```python
from build123d import *

# Parameters (mm, degrees)
F0_W      = 8
F0_H      = 5
F1_DEPTH  = 5
F2_R      = 0.75
F3_DEPTH  = 2
F4_W      = 4
F4_H      = 1.5
F5_DEPTH  = 23.5
F7_DEPTH  = 1.5
F8_W      = 1
F8_H      = 4
F9_DEPTH  = 30
F10_W     = 1
F10_H     = 2
F11_DEPTH = 1.5
F12_R     = 5
F13_DEPTH = 1
F15_ANGLE = 180
F16_R     = 0.49999
F17_R     = 0.5
F18_R     = 0.5


# Not quite as in the source:
# - a fillet or chamfer is up to 0.001 mm smaller than in the source, because OpenCascade refuses the exact size
# - a feature names something its author has since deleted; it is built from what else it names


with BuildPart() as f1:
    # F0 (on Front) → F1 (new body)
    with BuildSketch(Plane.XZ):
        Rectangle(F0_W, F0_H)
    extrude(amount=F1_DEPTH)

    # F2 (on face) → F3 (join)
    with BuildSketch(Plane.XZ.offset(5)):
        with Locations((-3, 1.5)):
            Circle(F2_R)
        with Locations((3, 1.5)):
            Circle(F2_R)
        with Locations((-3, -1.5)):
            Circle(F2_R)
        with Locations((3, -1.5)):
            Circle(F2_R)
    extrude(amount=F3_DEPTH)

    # F4 (on face) → F5 (join)
    with BuildSketch(Plane.XY.offset(2.5)):
        with Locations((0, -0.75)):
            Rectangle(F4_W, F4_H)
    extrude(amount=F5_DEPTH)

    # F6 (on face) → F7 (join)
    with BuildSketch(Plane(origin=(0, 0, 0), x_dir=(-1, 0, 0), z_dir=(0, 1, 0))):
        with BuildLine():
            ThreePointArc((2, 19.876524617), (4.5414755311, 21.8975815885), (5.5, 25))
            ThreePointArc((5.5, 25), (-3.1024184115, 29.5414755311), (-2, 19.876524617))
            Line((-2, 19.876524617), (-2, 26))
            Line((-2, 26), (2, 26))
            Line((2, 26), (2, 19.876524617))
        make_face()
        with BuildLine():
            Line((-2, 26), (-2, 19.876524617))
            ThreePointArc((-2, 19.876524617), (0, 19.5), (2, 19.876524617))
            Line((2, 19.876524617), (2, 26))
            Line((2, 26), (-2, 26))
        make_face()
    extrude(amount=-F7_DEPTH)

    # F8 (on face) → F9 (join)
    with BuildSketch(Plane.XZ.offset(1.5)):
        with Locations((0, 25)):
            Rectangle(F8_W, F8_H)
    extrude(amount=F9_DEPTH)

    # F10 (on face) → F11 (join)
    with BuildSketch(Plane.XZ.offset(31.5)):
        with Locations((0, 25)):
            Rectangle(F10_W, F10_H)
    extrude(amount=F11_DEPTH)

    # F12 (on face) → F13 (join)
    with BuildSketch(Plane(origin=(0, 0, 0), x_dir=(-1, 0, 0), z_dir=(0, 1, 0))):
        with Locations((0, 25)):
            Circle(F12_R)
    extrude(amount=F13_DEPTH)

    # F14 (on face) → F15 (revolve)
    with BuildSketch(Plane(origin=(0, 1, 0), x_dir=(-1, 0, 0), z_dir=(0, 1, 0))):
        with BuildLine():
            Line((0, 20), (0, 30))
            ThreePointArc((0, 30), (-5, 25), (0, 20))
        make_face()
    revolve(axis=Axis((0, 1, 25), (0, 0, 1)), revolution_arc=F15_ANGLE)

    # F16 (radius 0.5 in the source; OpenCascade refuses exactly that, so slightly less here)
    f16_edges = [f1.edges().sort_by_distance(p)[0] for p in [
        (-0.5, -16.5, 27),
        (0.5, -16.5, 27),
        (0.5, -16.5, 23),
        (-0.5, -16.5, 23),
    ]]
    fillet(f16_edges, radius=F16_R)

    # F17
    f17_edges = [f1.edges().sort_by_distance(p)[0] for p in [
        (-4, -2.5, 2.5),
        (-4, -2.5, -2.5),
        (4, -2.5, -2.5),
        (4, -2.5, 2.5),
    ]]
    fillet(f17_edges, radius=F17_R)

    # F18
    f18_edges = [f1.edges().sort_by_distance(p)[0] for p in [
        (-2, -1.5, 11.188262),
        (2, -1.5, 11.188262),
        (0, -1.5, 30.5),
    ]]
    fillet(f18_edges, radius=F18_R)


solid = f1.part
```
Model file for the job. Use its own axes, mm. A direction names the side the tool comes from. Coordinates: 2 decimals unless noted, no trailing zeros. Loops run counter-clockwise (first coordinate to the right, second up) from the corner with the lowest first, then second, coordinate; pieces in that order, holes last. Notation, with made-up numbers: (-3, 73) -> (20, 73) arc R23 ccw to (20, 84) -> close; hole circle Ø9 at (-22, 24.5). An arc over 180 degrees is marked (long way). Answer as a JSON object with one key per item and string values.
Q1. Pull direction Z, two halves, no side cores. Call faces 5 (the flat face through (0, -32, 24)), 6 (the flat face through (0, -5, 0)), 7 (the flat face through (-3, -7, -1)): released by +Z, released by -Z, zero draft, split by the parting line, or undercut.
Report:
{"face 5": "released by -Z", "face 6": "undercut", "face 7": "zero draft"}
Q2. Cut at D-D (z = -1.5). List the corners of the cut face in (x, y).
Report:
{"outline": "(-4, -5) -> (-3.75, -5) -> (-3.75, -7) -> (-2.25, -7) -> (-2.25, -5) -> (2.25, -5) -> (2.25, -7) -> (3.75, -7) -> (3.75, -5) -> (4, -5) -> (4, 0) -> (-4, 0) -> close"}
Q3. Cut at C-C (z = 16). List the corners of the cut face in (x, y).
Report:
{"outline": "(-2, -1) arc R0.5 ccw to (-1.5, -1.5) -> (1.5, -1.5) arc R0.5 ccw to (2, -1) -> (2, 0) -> (-2, 0) -> close"}
Q4. Probe probe 1 along X at (y, z) = (-26, 25); probe 2 along Y at (x, z) = (0.5, 16); probe 3 along X at (y, z) = (-1, 19.5). List the from-to ranges inside material, lowest first.
Report:
{"probe 1": "x = -0.5 to 0.5", "probe 2": "y = -1.5 to 0", "probe 3": "x = -2 to 2"}
Q5. Flat gauge pins, fed straight in: P1, Ø0.5, axis at y = -0.5, z = 10.5, coming from the -X side; P2, Ø4, axis at x = 0, y = -16.5, coming from the -Z side; P3, Ø0.8, axis at x = 0, z = 26.5, coming from the -Y side. Where does each tip first touch, or does it go through?
Report:
{"P1": "stops at x = -2", "P2": "stops at z = 23", "P3": "stops at y = -31.5"}
Q6. 3-axis set-ups, long thin cutter, end or side, ignore diameter. For faces 1 (the flat face through (4, -2, 0)), 2 (the flat face through (2, -0.5, 11.1)), 3 (the flat face through (-4, -2, 0)), 4 (the cylindrical face through (-3.595, -5.986, 1.044)): which of +Z, -Z, +X, -X, +Y, -Y reach the whole face in a straight line?
Report:
{"face 1": "-Z, +X, +Y, -Y", "face 2": "+X, +Y, -Y", "face 3": "-Z, -X, +Y, -Y", "face 4": "-Y"}
